Geometry: final body of the model. Coordinates: model frame, mm. Face numbers are marked on the shaded views. Give positions to 0.01 mm unless a question says otherwise; leave off trailing zeros. Loops run counter-clockwise (first coordinate to the right, second up) from the corner with the lowest first, then second, coordinate; pieces in that order, holes last.
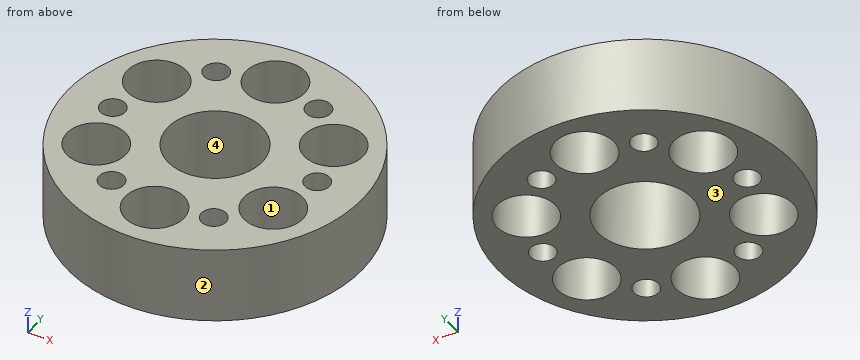
from build123d import *

# Parameters (mm, degrees)
SKETCH_1_R      = 25
SKETCH_1_R_2    = 8
SKETCH_1_R_3    = 2.1
SKETCH_1_R_4    = 5
EXTRUDE_2_DEPTH = 13


with BuildPart() as part:
    # 草图1 → 凸台-拉伸2 (new body)
    with BuildSketch(Plane.XY):
        with Locations(Location((0, 0, 0), (0, 0, 180))):
            Circle(SKETCH_1_R)
        with Locations(Location((0, 0, 0), (0, 0, 180))):
            Circle(SKETCH_1_R_2, mode=Mode.SUBTRACT)
        with Locations(Location((8.625, 14.938938215, 0), (0, 0, 180))):
            Circle(SKETCH_1_R_3, mode=Mode.SUBTRACT)
        with Locations(Location((17.25, 0, 0), (0, 0, 180))):
            Circle(SKETCH_1_R_3, mode=Mode.SUBTRACT)
        with Locations(Location((8.625, -14.938938215, 0), (0, 0, 180))):
            Circle(SKETCH_1_R_3, mode=Mode.SUBTRACT)
        with Locations(Location((-8.625, -14.938938215, 0), (0, 0, 180))):
            Circle(SKETCH_1_R_3, mode=Mode.SUBTRACT)
        with Locations(Location((-17.25, 0, 0), (0, 0, 180))):
            Circle(SKETCH_1_R_3, mode=Mode.SUBTRACT)
        with Locations(Location((-8.625, 14.938938215, 0), (0, 0, 180))):
            Circle(SKETCH_1_R_3, mode=Mode.SUBTRACT)
        with Locations(Location((0, 17.25, 0), (0, 0, 180))):
            Circle(SKETCH_1_R_4, mode=Mode.SUBTRACT)
        with Locations(Location((14.938938215, 8.625, 0), (0, 0, 180))):
            Circle(SKETCH_1_R_4, mode=Mode.SUBTRACT)
        with Locations(Location((14.938938215, -8.625, 0), (0, 0, 180))):
            Circle(SKETCH_1_R_4, mode=Mode.SUBTRACT)
        with Locations(Location((-14.938938215, -8.625, 0), (0, 0, 180))):
            Circle(SKETCH_1_R_4, mode=Mode.SUBTRACT)
        with Locations(Location((-14.938938215, 8.625, 0), (0, 0, 180))):
            Circle(SKETCH_1_R_4, mode=Mode.SUBTRACT)
        with Locations(Location((0, -17.25, 0), (0, 0, 180))):
            Circle(SKETCH_1_R_4, mode=Mode.SUBTRACT)
    extrude(amount=EXTRUDE_2_DEPTH)


solid = part.part
Item 1: Ray query, probe 1 along X at (y, z) = (-15.5, 9); probe 2 along Y at (x, z) = (2, 2); probe 3 along Y at (x, z) = (-16, 1.5). Return the intervals inside material, ascending.
Values follow:
probe 1: x = -19.62 to -10.65, -6.6 to -4.68, 4.68 to 6.6, 10.65 to 19.62
probe 2: y = -24.92 to -21.83, -12.67 to -7.75, 7.75 to 12.67, 21.83 to 24.92
probe 3: y = -19.21 to -13.51, -3.74 to -1.69, 1.69 to 3.74, 13.51 to 19.21
Item 2: Section query B-B on z = 4. Give the number of separate pieces and of enclosed holes in the cut face, plus the area to 3 significant figures.
Values follow:
separate pieces: 1
enclosed holes: 13
area: 1,210 mm2
Item 3: Section query C-C on y = 21. Return loops of the section in (x, z).
Values follow:
outline: (-13.56, 0) - (-3.31, 0) - (-3.31, 13) - (-13.56, 13) - close; (3.31, 0) - (13.56, 0) - (13.56, 13) - (3.31, 13) - close
Item 4: Section query A-A on y = 0. Return loops of the section in (x, z), plus the area to 3 significant figures.
Values follow:
outline: (-25, 0) - (-19.35, 0) - (-19.35, 13) - (-25, 13) - close; (-15.15, 0) - (-8, 0) - (-8, 13) - (-15.15, 13) - close; (8, 0) - (15.15, 0) - (15.15, 13) - (8, 13) - close; (19.35, 0) - (25, 0) - (25, 13) - (19.35, 13) - close
area: 333 mm2
Item 5: Pin query (flat end, axial travel): pin 1 (2.5 mm diameter, centred on x = 8.62, y = 14.94, fed in from +Z); pin 2 (5 mm diameter, centred on x = -0.5, z = 3.5, fed in from +Y); pin 3 (3 mm diameter, centred on x = -6.5, z = 10.5, fed in from +Y); pin 4 (3 mm diameter, centred on y = 17.5, z = 2, fed in from +X). Return the tip coordinate at first contact, or that it passes through.
Values follow:
pin 1: passes through
pin 2: stops at y = 25
pin 3: stops at y = 24.49
pin 4: stops at x = 19.21
Item 6: Draft query along Y for the marked faces 1, 2, 3 and 4. Return one class per face: +Y half, -Y half, draft (parallel to the pull), parting line (faces both ways), or undercut.
Values follow:
face 1: undercut
face 2: parting line
face 3: draft
face 4: undercut
Item 7: Section query D-D on x = -14.5. Return loops of the section in (y, z), plus the area to 3 significant figures.
Values follow:
outline: (-20.37, 0) - (-13.61, 0) - (-13.61, 13) - (-20.37, 13) - close; (-3.64, 0) - (3.64, 0) - (3.64, 13) - (-3.64, 13) - close; (13.61, 0) - (20.37, 0) - (20.37, 13) - (13.61, 13) - close
area: 271 mm2
